Autodesk Inventor part; units mm, degrees
ref_plane "YZ Plane" through (0, 0, 0) normal (1, 0, 0) x (0, 1, 0)
ref_plane "XZ Plane" through (0, 0, 0) normal (0, 1, 0) x (-1, 0, 0)
ref_plane "XY Plane" through (0, 0, 0) normal (0, 0, 1) x (1, 0, 0)
sketch "Эскиз2" plane through (0, 0, 0) normal (0, 0, 1) x (1, 0, 0)
  circle A0 centre (0, 0) radius 107.5
  circle A1 centre (0, 0) radius 104
  line L0 (-99.2724, 31) -> (-78.7724, 31)
  line L1 (-99.2724, -31) -> (-78.7724, -31)
  line L2 (-31, 99.2724) -> (-31, 78.7724)
  line L3 (31, 99.2724) -> (31, 78.7724)
  line L4 (99.2724, 31) -> (78.7724, 31)
  line L5 (99.2724, -31) -> (78.7724, -31)
  line L6 (31, -99.2724) -> (31, -78.7724)
  line L7 (-31, -99.2724) -> (-31, -78.7724)
  line L8 (-78.7724, -31) -> (-78.7724, 31)
  line L9 (-31, 78.7724) -> (31, 78.7724)
  line L10 (78.7724, 31) -> (78.7724, -31)
  line L11 (31, -78.7724) -> (-31, -78.7724)
  circle A2 centre (-109.0212, -109.0212) radius 75.25
  line L12 (-31, 78.7724) -> (78.7724, -31) construction
  line L13 (-73.5391, 73.5391) -> (73.5391, -73.5391) construction
  circle A3 centre (109.0212, 109.0212) radius 75.25
  point P0 (-98.0863, -34.57)
  point P1 (-34.57, -98.0863)
  point P2 (98.0863, 34.57)
  point P3 (34.57, 98.0863)
  dimension "d1" = 208
  dimension "d0" = 215
  dimension "d8" = 20.5
  dimension "d9" = 31
  dimension "d10" = 31
  dimension "d11" = 31
  dimension "d12" = 31
  dimension "d13" = 31
  dimension "d14" = 31
  dimension "d15" = 31
  dimension "d16" = 31
  dimension "d17" = 150.5
  dimension "d18" = 3.57
  dimension "d19" = 3.57
extrude "Выдавливание1" add sketch "Эскиз2" along normal blind 3 contours A1 L4 L10 L5 L6 L11 L7 A2 L1 L8 L0 L2 L9 L3 A3
sketch "Эскиз3" plane through (0, 0, 0) normal (0, 0, -1) x (-1, 0, 0)
  line L0 (-78.7724, -31) -> (-78.7724, 31)
  line L1 (-78.7724, 16) -> (78.7724, 16) construction
  line L2 (78.7724, 31) -> (78.7724, -31)
  line L3 (-31, 78.7724) -> (31, 78.7724)
  line L4 (31, -78.7724) -> (-31, -78.7724)
  line L5 (-16, -78.7724) -> (-16, 78.7724) construction
  line L6 (0, 0) -> (0, 78.7724) construction
  line L7 (0, 0) -> (78.7724, 0) construction
  line L8 (-78.7724, -16) -> (78.7724, -16) construction
  line L9 (16, -78.7724) -> (16, 78.7724) construction
  circle A0 centre (-49.72, 16) radius 1.5
  circle A1 centre (-49.72, -16) radius 1.5
  circle A2 centre (-16, 49.72) radius 1.5
  circle A3 centre (16, 49.72) radius 1.5
  circle A4 centre (49.72, 16) radius 1.5
  circle A5 centre (49.72, -16) radius 1.5
  line L10 (-49.72, 49.72) -> (49.72, 49.72) construction
  line L11 (49.72, 49.72) -> (49.72, -49.72) construction
  line L12 (49.72, -49.72) -> (-49.72, -49.72) construction
  line L13 (-49.72, -49.72) -> (-49.72, 49.72) construction
  line L14 (-49.72, 49.72) -> (49.72, -49.72) construction
  circle A6 centre (-16, -49.72) radius 1.5
  circle A7 centre (16, -49.72) radius 1.5
  line L15 (-72.43, 72.43) -> (72.43, 72.43) construction
  line L16 (72.43, 72.43) -> (72.43, -72.43) construction
  line L17 (72.43, -72.43) -> (-72.43, -72.43) construction
  line L18 (-72.43, -72.43) -> (-72.43, 72.43) construction
  line L19 (-72.43, 72.43) -> (72.43, -72.43) construction
  circle A8 centre (-72.43, 16) radius 1.5
  circle A9 centre (-72.43, -16) radius 1.5
  circle A10 centre (-16, 72.43) radius 1.5
  circle A11 centre (16, 72.43) radius 1.5
  circle A12 centre (72.43, 16) radius 1.5
  circle A13 centre (72.43, -16) radius 1.5
  circle A14 centre (16, -72.43) radius 1.5
  circle A15 centre (-16, -72.43) radius 1.5
  circle A16 centre (-72.43, 31) radius 1.5
  circle A17 centre (-31, 72.43) radius 1.5
  circle A18 centre (31, -72.43) radius 1.5
  circle A19 centre (72.43, -31) radius 1.5
  line L20 (-99.2724, -31) -> (-78.7724, -31)
  line L21 (-31, -78.7724) -> (-31, -99.2724)
  arc A20 (-89.0224, -31) -> (-31, -89.0224) centre (0, 0) ccw construction
  arc A21 (89.0224, 31) -> (31, 89.0224) centre (0, 0) ccw construction
  circle A22 centre (-57.67, -74.5664) radius 1.5
  line L22 (-72.43, -72.43) -> (72.43, 72.43) construction
  circle A23 centre (-74.5664, -57.67) radius 1.5
  circle A24 centre (-44.87, -82.9015) radius 1.5
  circle A25 centre (-82.9015, -44.87) radius 1.5
  circle A26 centre (74.5664, 57.67) radius 1.5
  circle A27 centre (57.67, 74.5664) radius 1.5
  circle A28 centre (82.9015, 44.87) radius 1.5
  circle A29 centre (44.87, 82.9015) radius 1.5
  arc A30 (-98.0863, 34.57) -> (-34.57, 98.0863) centre (-109.0212, 109.0212) ccw
  dimension "d22" = 16
  dimension "d23" = 16
  dimension "d25" = 99.44
  dimension "d26" = 3
  dimension "d27" = 144.86
  dimension "d28" = 3
  dimension "d29" = 3
  dimension "d30" = 15
  dimension "d31" = 15
  dimension "d32" = 15
  dimension "d33" = 15
  dimension "d35" = 26.67
  dimension "d36" = 13.87
  dimension "d37" = 3
extrude "Выдавливание2" cut sketch "Эскиз3" against normal blind 3
properties part number "floor"
Read the model definition and answer for the solid it produces. Units are mm, in the model's axes. Give positions to 0.01 mm unless a question says otherwise; leave off trailing zeros. Use CSV: the item, a comma, the result in double quotes. Start each with the question number.
(1) Find section A-A (z = 1.3). Count the separate pieces of the cut face and the enclosed holes in it, plus the area to 3 significant figures.
(2) Given P1, Ø1.5, axis at y = -50, z = 2.5, coming from the -X side; P2, Ø0.9, axis at x = 85, z = 1.5, coming from the +Y side; P3, Ø1, axis at x = -56, z = 2.5, coming from the -Y side, each flat-ended and moving along its own axis, determine where each tip first touches the part or whether it passes through.
(3) Consider line 1 along Y through (x, z) = (-16, 1.4); line 2 along X through (y, z) = (72.43, 1.45); line 3 along Y through (x, z) = (-72, 2.2). Determine where each line is inside the solid, lowest interval first.
Findings below:
1,separate pieces,"1"
1,enclosed holes,"28"
1,area,"24,900 mm2"
2,P1,"x = -63.31"
2,P2,"y = 37.86"
2,P3,"y = -56.12"
3,line 1,"-78.77 to -73.93, -70.93 to -51.22, -48.22 to 48.22, 51.22 to 70.93, 73.93 to 78.77"
3,line 2,"-74.63 to -17.5, -14.5 to 14.5, 17.5 to 29.5, 32.5 to 43.27"
3,line 3,"-43.51 to -32.44, -29.56 to -17.44, -14.56 to 14.56, 17.44 to 75.05"
